from build123d import *

# Parameters (mm, degrees)
F0_R     = 9.525
F1_DEPTH = 25.4
F3_DEPTH = 25.401
F4_DEPTH = 8.636
F6_DEPTH = 9.525


with BuildPart() as f1:
    # F0 (on Front) → F1 (new body)
    with BuildSketch(Plane.XZ):
        Circle(F0_R)
    extrude(amount=F1_DEPTH)

    # F2 (on Front) → F3 (cut, through all)
    with BuildSketch(Plane.XZ):
        with BuildLine():
            ThreePointArc((4.7625, 0), (3.367596, 3.367596), (0, 4.7625))
            ThreePointArc((0, 4.7625), (-3.367596, 3.367596), (-4.7625, 0))
            ThreePointArc((-4.7625, 0), (-3.367596, -3.367596), (0, -4.7625))
            ThreePointArc((0, -4.7625), (3.367596, -3.367596), (4.7625, 0))
        make_face()
    extrude(amount=F3_DEPTH, mode=Mode.SUBTRACT)

    # F2 (on Front) → F4 (cut)
    with BuildSketch(Plane.XZ):
        with BuildLine():
            ThreePointArc((-4.7625, 0), (-3.367596, 3.367596), (0, 4.7625))
            Line((0, 4.7625), (-4.7625, 4.7625))
            Line((-4.7625, 4.7625), (-4.7625, 0))
        make_face()
        with BuildLine():
            Line((4.7625, 0), (4.7625, 4.7625))
            Line((4.7625, 4.7625), (0, 4.7625))
            ThreePointArc((0, 4.7625), (3.367596, 3.367596), (4.7625, 0))
        make_face()
        with BuildLine():
            ThreePointArc((0, -4.7625), (-3.367596, -3.367596), (-4.7625, 0))
            Line((-4.7625, 0), (-4.7625, -4.7625))
            Line((-4.7625, -4.7625), (0, -4.7625))
        make_face()
        with BuildLine():
            Line((4.7625, -4.7625), (4.7625, 0))
            ThreePointArc((4.7625, 0), (3.367596, -3.367596), (0, -4.7625))
            Line((0, -4.7625), (4.7625, -4.7625))
        make_face()
    extrude(amount=F4_DEPTH, mode=Mode.SUBTRACT)

    # F5 (on face) → F6 (cut)
    with BuildSketch(Plane.XZ.offset(25.4)):
        Polygon((3.65125, 6.324151), (-3.65125, 6.324151), (-7.3025, 0), (-3.65125, -6.324151), (3.65125, -6.324151), (7.3025, 0), align=None)
    extrude(amount=-F6_DEPTH, mode=Mode.SUBTRACT)


solid = f1.part
Geometry: final body of the model. Coordinates: model frame, mm. A direction names the side the tool comes from. Coordinates: 2 decimals unless noted, no trailing zeros. Order: outer loops, then holes, each group sorted by start corner. A loop starts at its lowest first (then second) coordinate and runs counter-clockwise, first axis right, second up.
(1) Access query for faces 1 (the face through (6.2, -25.4, 2.3)), 2 (the face through (5, -15.875, 0)), 3 (the face through (0, -4, 4.762)). Directions: +Z, -Z, +X, -X, +Y, -Y. A direction counts if a zero-diameter tool reaches every point of the face in a straight line with its end or side. Return the directions, or none.
(2) First-contact query: pin 1 (2 mm diameter, centred on y = -12, z = -7.5, fed in from +X); pin 2 (1.5 mm diameter, centred on y = -13, z = -7.5, fed in from -X); pin 3 (6.5 mm diameter, centred on x = 2, z = 2, fed in from -Y) (3 decimals). Flat tips, straight axial feed; report the tip coordinate or a pass-through.
(3) Material intervals for probe 1 along Z at (x, y) = (0.25, -6.25); probe 2 along Y at (x, z) = (5.5, -1.25) (3 decimals); probe 3 along X at (y, z) = (-19.25, 5), sorted ascending.
(4) Section query A-A (x = -2.75). Return the cut outline in (y, z) (1 decimal), plus the area to 3 significant figures.
(5) Draft query along X for faces 4 (the face through (0, -4, -4.762)), 5 (the face through (-7.559, -12.522, -5.796)), 6 (the face through (-4.762, -4, 0)), 7 (the face through (0, 0, -6)). Return one class per face: pulls with the +X half, pulls with the -X half, needs draft (parallel to the pull), parting line crosses it, or undercut.
Solution:
1. face 1: +Z, -Z, +X, -X, -Y
1. face 2: -Y
1. face 3: +Y
2. pin 1: stops at x = 6.96
2. pin 2: stops at x = -6.72
2. pin 3: stops at y = -15.875
3. probe 1: z = -9.52 to -4.76, 4.76 to 9.52
3. probe 2: y = -15.875 to 0
3. probe 3: x = -8.11 to -4.42, 4.42 to 8.11
4. outline: (-25.4, -9.1) - (0, -9.1) - (0, -4.8) - (-8.6, -4.8) - (-8.6, -3.9) - (-15.9, -3.9) - (-15.9, -6.3) - (-25.4, -6.3) - close; (-25.4, 6.3) - (-15.9, 6.3) - (-15.9, 3.9) - (-8.6, 3.9) - (-8.6, 4.8) - (0, 4.8) - (0, 9.1) - (-25.4, 9.1) - close
4. area: 204 mm2
5. face 4: undercut
5. face 5: parting line crosses it
5. face 6: undercut
5. face 7: needs draft
